For this review, use the dimensioned drawing (mm, ordinates from the lowest corner) and the shaded views. Give positions to 0.01 mm unless a question says otherwise; leave off trailing zeros. Order: outer loops, then holes, each group sorted by start corner. A loop starts at its lowest first (then second) coordinate and runs counter-clockwise, first axis right, second up. Notation, with made-up numbers: M 13.5,30 L 65.5,30 A11 cw 65.5,40 Z; hole C -13,6 d8. An arc over 180 degrees is marked long. One line per question, with ' | ' between items. Start each with the question number.
1. We need section D-D on x = 51.5. Write out the cut boundary in (y, z) (1 decimal).
2. Insertion check: P1, Ø1, axis at y = 14, z = 2, coming from the -X side; P2, Ø1.6, axis at x = 63.5, z = 2.5, coming from the -Y side. Each pin has a flat end and moves straight along its axis. Give the tip position at first contact, or say it passes through.
3. We need section C-C on y = 9. Write out the cut boundary in (x, z) (1 decimal).
4. Wall thickness on L1, parallel to Y at x = 40.5, z = 2.6 (1 decimal); L2, parallel to X at y = 10, z = 2.7 (1 decimal); L3, parallel to Y at x = 4, z = 1.9 (1 decimal): over which ranges is each line inside the solid? List them lowest first.
5. We need section B-B on z = 2.1. Write out the cut boundary in (x, y) (1 decimal), then the cut area to 3 significant figures.
6. We need section A-A on x = 38. Write out the cut boundary in (y, z) (1 decimal).
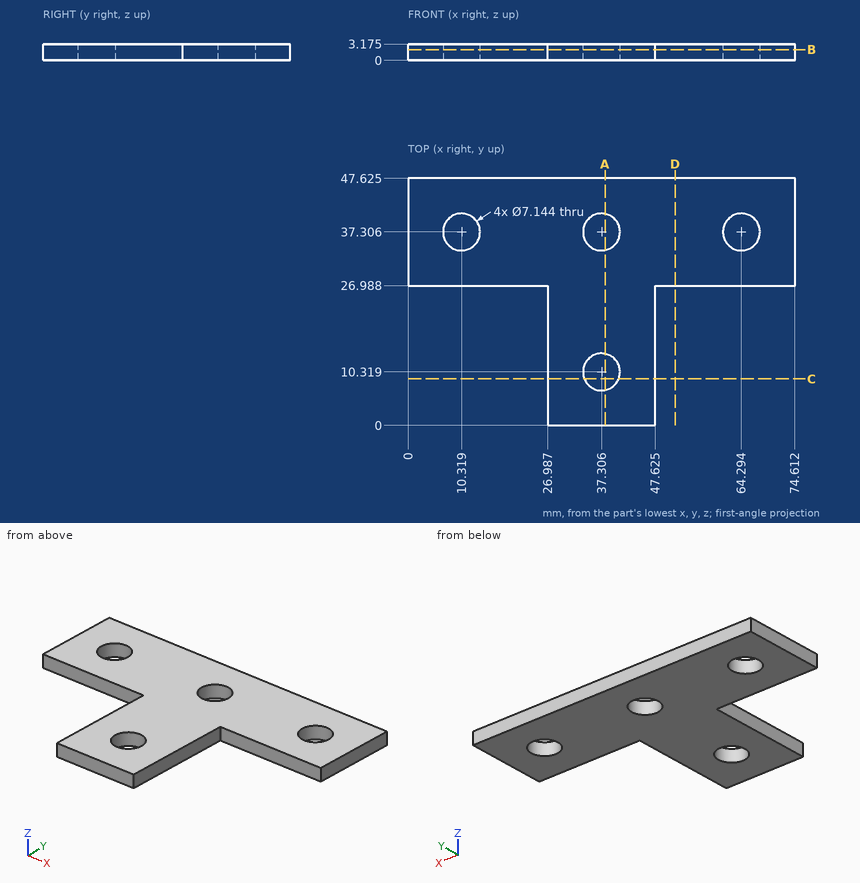
Entries:
1) outline: M 27,0 L 47.6,0 L 47.6,3.2 L 27,3.2 Z
2) P1: stops at x = 26.99 | P2: stops at y = 26.99
3) outline: M 27,0 L 34,0 L 34,3.2 L 27,3.2 Z; M 40.6,0 L 47.6,0 L 47.6,3.2 L 40.6,3.2 Z
4) L1: y = 0 to 8.7, 11.9 to 35.7, 38.9 to 47.6 | L2: x = 27 to 33.7, 40.9 to 47.6 | L3: y = 27 to 47.6
5) outline: M 0,27 L 27,27 L 27,0 L 47.6,0 L 47.6,27 L 74.6,27 L 74.6,47.6 L 0,47.6 Z; hole C 10.3,37.3 d7.1; hole C 37.3,10.3 d7.1; hole C 37.3,37.3 d7.1; hole C 64.3,37.3 d7.1 | area: 1,940 mm^2
6) outline: M 0,0 L 6.8,0 L 6.8,3.2 L 0,3.2 Z; M 13.8,0 L 33.8,0 L 33.8,3.2 L 13.8,3.2 Z; M 40.8,0 L 47.6,0 L 47.6,3.2 L 40.8,3.2 Z
